Read the model definition and answer for the solid it produces. Units are mm, in the model's axes. A direction names the side the tool comes from. Coordinates: 2 decimals unless noted, no trailing zeros. Write each loop counter-clockwise with the first axis right and the second up, starting at its lowest first coordinate (ties: lowest second). Pieces come first, ordered by that corner, then holes. Notation, with made-up numbers: (30.5, 31.5) - (55.5, 31.5) arc R17 cw to (55.5, 36.5) - close; hole circle Ø4 at (-33.5, 40). An arc over 180 degrees is marked (long way). Return JSON: item names as keys, results as strings.
```python
from build123d import *

# Parameters (mm, degrees)
SKETCH2_R           = 14
BOSS_EXTRUDE1_DEPTH = 4
BOSS_EXTRUDE2_DEPTH = 2.5
BOSS_EXTRUDE3_DEPTH = 4
SKETCH5_R           = 14
BOSS_EXTRUDE4_DEPTH = 4
BOSS_EXTRUDE5_START = 2
SKETCH6_R           = 14
BOSS_EXTRUDE5_DEPTH = 2


with BuildPart() as part:
    # Sketch2 → Boss-Extrude1 (new body)
    with BuildSketch(Plane(origin=(0, 0, 0), x_dir=(0, 0, -1), z_dir=(1, 0, 0))):
        Circle(SKETCH2_R)
    extrude(amount=BOSS_EXTRUDE1_DEPTH)

    # Sketch3 → Boss-Extrude2 (add)
    with BuildSketch(Plane(origin=(4, 0, 0), x_dir=(0, 0, -1), z_dir=(1, 0, 0))):
        with BuildLine():
            Line((-35.15, 12.5), (-35.15, -12.5))
            Line((-35.15, -12.5), (-27.15, -12.5))
            Line((-27.15, -12.5), (-23.15, -10.555257391))
            Line((-23.15, -10.555257391), (-6.017394902, -10.555257391))
            ThreePointArc((-6.017394902, -10.555257391), (12.15, 0), (-6.017394902, 10.555257391))
            Line((-6.017394902, 10.555257391), (-23.15, 10.555257391))
            Line((-23.15, 10.555257391), (-27.15, 12.5))
            Line((-27.15, 12.5), (-35.15, 12.5))
        make_face()
    extrude(amount=BOSS_EXTRUDE2_DEPTH)

    # Sketch4 → Boss-Extrude3 (add)
    with BuildSketch(Plane.XY.offset(35.15)):
        with BuildLine():
            Line((12.5, -11.35), (29.791469844, -11.35))
            ThreePointArc((29.791469844, -11.35), (55.6, 0), (29.791469844, 11.35))
            Line((29.791469844, 11.35), (12.5, 11.35))
            Line((12.5, 11.35), (9.5, 12.5))
            Line((9.5, 12.5), (6.5, 12.5))
            Line((6.5, 12.5), (6.5, -12.5))
            Line((6.5, -12.5), (9.5, -12.5))
            Line((9.5, -12.5), (12.5, -11.35))
        make_face()
    extrude(amount=-BOSS_EXTRUDE3_DEPTH)

    # Sketch5 → Boss-Extrude4 (add)
    with BuildSketch(Plane.XY.offset(35.15)):
        with Locations((40.2, 0)):
            Circle(SKETCH5_R)
    extrude(amount=BOSS_EXTRUDE4_DEPTH)

    # Sketch6 → Boss-Extrude5 (add)
    with BuildSketch(Plane(origin=(0, 0, 31.15), x_dir=(-1, 0, 0), z_dir=(0, 0, -1)).offset(BOSS_EXTRUDE5_START)):
        with Locations(Location((-40.2, 0, 0), (0, 0, 180))):
            Circle(SKETCH6_R)
    extrude(amount=-BOSS_EXTRUDE5_DEPTH)


solid = part.part
```
(1) A cutting plane is placed at A-A (z = 0). Determine the outline of the cut face in (x, y).
Answer:
{"outline": "(0, -14) - (4, -14) - (4, -12.15) - (6.5, -12.15) - (6.5, 12.15) - (4, 12.15) - (4, 14) - (0, 14) - close"}
(2) Straight lines are drawn through the part: line 1 (Z direction, x = 33.5, y = 4.5); line 2 (X direction, y = 5.5, z = -10); line 3 (X direction, y = 7.5, z = 12). For each, find the intervals that lie inside material, in ascending order. Write a range as from..to.
Answer:
{"line 1": "29.15..39.15", "line 2": "0..6.5", "line 3": "4..6.5"}
(3) A cutting plane is placed at C-C (y = 0). Determine the outline of the cut face in (x, z), and give its area (3 significant figures).
Answer:
{"outline": "(0, -14) - (4, -14) - (4, -12.15) - (6.5, -12.15) - (6.5, 31.15) - (26.2, 31.15) - (26.2, 29.15) - (54.2, 29.15) - (54.2, 31.15) - (55.6, 31.15) - (55.6, 35.15) - (54.2, 35.15) - (54.2, 39.15) - (26.2, 39.15) - (26.2, 35.15) - (4, 35.15) - (4, 14) - (0, 14) - close", "area": "595 mm²"}
(4) Which of the six approach directions +Z, -Z, +X, -X, +Y, -Y give full straight-line access (tool end or side, diameter ignored) to faces 1 (the face through (5.232, -0.355, -12.145)), 2 (the face through (5.232, 11.514, 25.122)), 3 (the face through (11.021, 11.917, 33.178)), 4 (the face through (21, -11.35, 33))?
Answer:
{"face 1": "+X", "face 2": "+X, -X, +Y", "face 3": "+Z, -Z, +Y", "face 4": "+Z, -Z, -Y"}
(5) Flat-ended cylindrical pins translate along their axes: P1, Ø1.6, axis at x = 6.5, z = 32.5, coming from the +Y side; P2, Ø1.6, axis at x = 7, z = 30.5, coming from the -Y side; P3, Ø0.8, axis at x = 6, z = 13.5, coming from the +Y side. Find the tip coordinate at first contact, or state that the pin passes through.
Answer:
{"P1": "y = 12.5", "P2": "y = -12.5", "P3": "y = 10.56"}
(6) A cutting plane is placed at D-D (z = 13). Determine the outline of the cut face in (x, y), and give its area (3 significant figures).
Answer:
{"outline": "(0, -5.2) - (4, -5.2) - (4, -10.56) - (6.5, -10.56) - (6.5, 10.56) - (4, 10.56) - (4, 5.2) - (0, 5.2) - close", "area": "94.3 mm²"}
(7) Determine the mould class of faces 5 (the face through (0, 0, 0)), 6 (the face through (5, -10.555, 15)), 7 (the face through (40, 0, 29.15)), 8 (the face through (1.972, -5.362, -12.932)) for opening direction Z: +Z half, -Z half, draft (parallel to the pull), parting line (faces both ways), or undercut.
Answer:
{"face 5": "draft", "face 6": "undercut", "face 7": "-Z half", "face 8": "parting line"}
(8) A cutting plane is placed at B-B (x = 40.2). Determine the outline of the cut face in (y, z).
Answer:
{"outline": "(-15.4, 31.15) - (-14, 31.15) - (-14, 29.15) - (14, 29.15) - (14, 31.15) - (15.4, 31.15) - (15.4, 35.15) - (14, 35.15) - (14, 39.15) - (-14, 39.15) - (-14, 35.15) - (-15.4, 35.15) - close"}
